```python
from build123d import *

# Parameters (mm, degrees)
SKETCH_1_W          = 34
SKETCH_1_H          = 49
EXTRUDE_1_DEPTH     = 10
SKETCH_2_W          = 1.5
SKETCH_2_H          = 24
EXTRUDE_2_DEPTH     = 4
SKETCH_3_W          = 1.5
SKETCH_3_H          = 12
SKETCH_3_W_2        = 25
SKETCH_3_H_2        = 13
CUT_EXTRUDE_1_DEPTH = 10
SKETCH_4_R          = 2
CUT_EXTRUDE_2_DEPTH = 31
EXTRUDE_3_DEPTH     = 8
CUT_EXTRUDE_4_DEPTH = 10
SKETCH_6_W          = 16
SKETCH_6_H          = 25
EXTRUDE_4_DEPTH     = 3
SKETCH_7_R          = 1.65
CUT_EXTRUDE_5_DEPTH = 8


with BuildPart() as part:
    # 草图1 → 凸台-拉伸1 (new body)
    with BuildSketch(Plane(origin=(0, 0, 0), x_dir=(1, 0, 0), z_dir=(0, 1, 0))):
        Rectangle(SKETCH_1_W, SKETCH_1_H)
    extrude(amount=EXTRUDE_1_DEPTH)

    # 草图2 → 凸台-拉伸2 (add)
    with BuildSketch(Plane(origin=(0, 10, 0), x_dir=(1, 0, 0), z_dir=(0, 1, 0))):
        with Locations((-16.25, 7.5)):
            Rectangle(SKETCH_2_W, SKETCH_2_H)
        with Locations((16.25, 7.5)):
            Rectangle(SKETCH_2_W, SKETCH_2_H)
    extrude(amount=EXTRUDE_2_DEPTH)

    # 草图3 → 切除-拉伸1 (cut)
    with BuildSketch(Plane(origin=(0, 10, 0), x_dir=(1, 0, 0), z_dir=(0, 1, 0))):
        with Locations((-16.25, -18.5)):
            Rectangle(SKETCH_3_W, SKETCH_3_H)
        with Locations((16.25, -18.5)):
            Rectangle(SKETCH_3_W, SKETCH_3_H)
        with Locations((0, -18)):
            Rectangle(SKETCH_3_W_2, SKETCH_3_H_2)
    extrude(amount=-CUT_EXTRUDE_1_DEPTH, mode=Mode.SUBTRACT)

    # 草图4 → 切除-拉伸2 (cut)
    with BuildSketch(Plane.ZY.offset(15.5)):
        with Locations((18.5, 6)):
            Circle(SKETCH_4_R)
    extrude(amount=-CUT_EXTRUDE_2_DEPTH, mode=Mode.SUBTRACT)

    # 草图5 → 凸台-拉伸3 (add)
    with BuildSketch(Plane.XZ):
        Polygon((4, 11.5), (-4, 11.5), (-4, 41.5), (-13, 41.5), (-13, 56.5), (13, 56.5), (13, 41.5), (4, 41.5), align=None)
    extrude(amount=-EXTRUDE_3_DEPTH)

    # 草图5<2> → 切除-拉伸4 (cut)
    with BuildSketch(Plane.XZ):
        Polygon((4, 11.5), (-4, 11.5), (-4, 41.5), (-13, 41.5), (-13, 56.5), (13, 56.5), (13, 41.5), (4, 41.5), align=None)
    extrude(amount=-CUT_EXTRUDE_4_DEPTH, mode=Mode.SUBTRACT)

    # 草图6 → 凸台-拉伸4 (add)
    with BuildSketch(Plane.XZ):
        with Locations((25, -6)):
            Rectangle(SKETCH_6_W, SKETCH_6_H)
        with Locations((-25, -6)):
            Rectangle(SKETCH_6_W, SKETCH_6_H)
    extrude(amount=-EXTRUDE_4_DEPTH)

    # 草图7 → 切除-拉伸5 (cut)
    with BuildSketch(Plane.XZ):
        with Locations((29.112405101, 1.5)):
            Circle(SKETCH_7_R)
        with Locations((29.112405101, -10.5)):
            Circle(SKETCH_7_R)
        with Locations((-29.887594899, 1.5)):
            Circle(SKETCH_7_R)
        with Locations((-29.887594899, -10.5)):
            Circle(SKETCH_7_R)
    extrude(amount=-CUT_EXTRUDE_5_DEPTH, mode=Mode.SUBTRACT)


solid = part.part
```
Source: CAD feature listing. Evaluate the final solid. Frame: model axes, mm. A direction names the side the tool comes from. Coordinates: 2 decimals unless noted, no trailing zeros. Write each loop counter-clockwise with the first axis right and the second up, starting at its lowest first coordinate (ties: lowest second). Pieces come first, ordered by that corner, then holes. Notation, with made-up numbers: M 40,29 L 62,29 A18 cw 62,61 Z; hole C -9.5,71 d3. An arc over 180 degrees is marked long. Answer as a JSON object with one key per item and string values.
1. Cut plane D-D on x = -13.5. Output: boundary loops of the cut face in (y, z), plus the area to 3 significant figures.
Evaluation:
{"outline": "M 0,-24.5 L 10,-24.5 L 10,24.5 L 0,24.5 Z; hole C 6,18.5 d4", "area": "477 mm^2"}
2. Cut plane A-A on y = 11.75. Output: boundary loops of the cut face in (x, z).
Evaluation:
{"outline": "M -17,-19.5 L -15.5,-19.5 L -15.5,4.5 L -17,4.5 Z; M 15.5,-19.5 L 17,-19.5 L 17,4.5 L 15.5,4.5 Z"}
3. Contact query for flat-ended pins moving along their axis: P1, Ø0.8, axis at x = 16.5, y = 11.5, coming from the -Z side; P2, Ø3, axis at y = 6.5, z = 19.5, coming from the +X side; P3, Ø6, axis at y = 5.5, z = 12.5, coming from the -X side. Output: stop coordinate, or through.
Evaluation:
{"P1": "z = -19.5", "P2": "x = 15.5", "P3": "x = -17"}
4. Access query for faces 1 (the flat face through (-12.5, 4, 17)), 2 (the flat face through (16, 12, -19.5)), 3 (the flat face through (-25, 3, -6)). Directions: +Z, -Z, +X, -X, +Y, -Y. A direction counts if a zero-diameter tool reaches every point of the face in a straight line with its end or side. Return the directions, or none.
Evaluation:
{"face 1": "+Z, +Y, -Y", "face 2": "-Z, +X, -X, +Y", "face 3": "+Z, -Z, -X, +Y"}
5. Draft query along Z for faces 4 (the flat face through (16, 14, -8)), 5 (the flat face through (16, 12, 4.5)), 6 (the cylindrical face through (-28.363, 1.479, -11.132)). Return one class per face: released by +Z, released by -Z, zero draft, split by the parting line, or undercut.
Evaluation:
{"face 4": "zero draft", "face 5": "released by +Z", "face 6": "undercut"}
6. Cut plane B-B on z = 18.5. Output: boundary loops of the cut face in (x, y).
Evaluation:
{"outline": "M -15.5,0 L -12.5,0 L -12.5,4 L -15.5,4 Z; M -15.5,8 L -12.5,8 L -12.5,10 L -15.5,10 Z; M 12.5,0 L 15.5,0 L 15.5,4 L 12.5,4 Z; M 12.5,8 L 15.5,8 L 15.5,10 L 12.5,10 Z"}
7. Ray query, L1, parallel to X at y = 12.75, z = 1; L2, parallel to Y at x = 14, z = -19; L3, parallel to X at y = 2.75, z = 9. Return the intervals inside material, ascending.
Evaluation:
{"L1": "-17 to -15.5, 15.5 to 17", "L2": "0 to 10", "L3": "-17 to 17"}
8. Cut plane C-C on z = -10.5. Output: boundary loops of the cut face in (x, y), plus the area to 3 significant figures.
Evaluation:
{"outline": "M -33,0 L -31.54,0 L -31.54,3 L -33,3 Z; M -28.24,0 L 27.46,0 L 27.46,3 L 17,3 L 17,14 L 15.5,14 L 15.5,10 L -15.5,10 L -15.5,14 L -17,14 L -17,3 L -28.24,3 Z; M 30.76,0 L 33,0 L 33,3 L 30.76,3 Z", "area": "428 mm^2"}
